Drawing for the job (mm, zero at the part's lowest x, y, z). A direction names the side the tool comes from. Give positions to 0.01 mm unless a question says otherwise; leave off trailing zeros. Loops run counter-clockwise (first coordinate to the right, second up) from the corner with the lowest first, then second, coordinate; pieces in that order, holes last.
1) Band-saw the part on A-A on z = 6.5. List the corners of the cut face in (x, y).
2) Band-saw the part on D-D on y = 35. List the corners of the cut face in (x, z).
3) 3-axis set-ups, long thin cutter, end or side, ignore diameter. For the marked faces 1 and 2: which of +Z, -Z, +X, -X, +Y, -Y reach the whole face in a straight line?
4) Flat gauge pins, fed straight in: P1, Ø3, axis at x = 38.5, y = 20, coming from the -Z side; P2, Ø1.6, axis at y = 10.91, z = 25.25, coming from the -X side. Where does each tip first touch, or does it go through?
5) Band-saw the part on B-B on x = 11.5. List the corners of the cut face in (y, z), then the cut area to 3 significant figures.
6) Wall check: line 1 (Y direction, x = 66.2, z = 14.75); line 2 (Z direction, x = 19, y = 2.5); line 3 (X direction, y = 7.5, z = 26). Give the ranges that are in metal, low to high.
7) Band-saw the part on C-C on y = 20. State how many separate pieces and enclosed holes the cut face has.
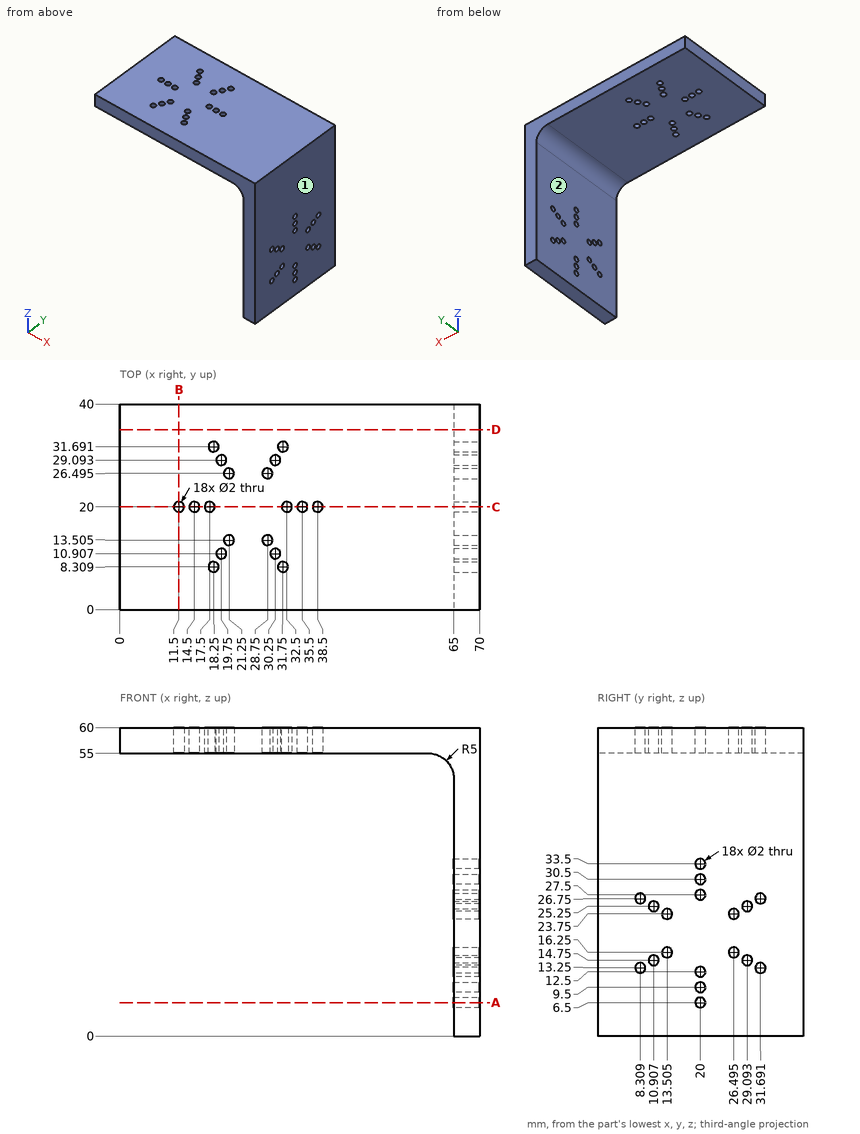
Findings below:
1. outline: (65, 0) - (70, 0) - (70, 19) - (65, 19) - close; (65, 21) - (70, 21) - (70, 40) - (65, 40) - close
2. outline: (0, 55) - (60, 55) arc R5 cw to (65, 50) - (65, 0) - (70, 0) - (70, 60) - (0, 60) - close
3. face 1: +Z, -Z, +X, +Y, -Y
3. face 2: -Z, -X, +Y, -Y
4. P1: stops at z = 55
4. P2: passes through
5. outline: (0, 55) - (19, 55) - (19, 60) - (0, 60) - close; (21, 55) - (40, 55) - (40, 60) - (21, 60) - close
5. area: 190 mm2
6. line 1: y = 0 to 9.91, 11.91 to 28.09, 30.09 to 40
6. line 2: z = 55 to 60
6. line 3: x = 65 to 70
7. separate pieces: 13
7. enclosed holes: 0
